Geometry: final body of the model. Coordinates: model frame, mm. Face numbers are marked on the shaded views. A direction names the side the tool comes from. Coordinates: 2 decimals unless noted, no trailing zeros. Order: outer loops, then holes, each group sorted by start corner. A loop starts at its lowest first (then second) coordinate and runs counter-clockwise, first axis right, second up. Notation, with made-up numbers: (2, -32) -> (49, -32) arc R28 cw to (49, -8) -> close; hole circle Ø2 at (-23, 16). An arc over 180 degrees is marked (long way). Answer in a Markdown table with one row per item. Add a question column.
1) Set-up query: the marked faces 1, 2, 3 and 4. Return all of +Z, -Z, +X, -X, +Y, -Y with unobstructed straight access to the full face (end or side cutting, diameter ignored); none if empty.
2) Ray query, line 1 (Y direction, x = -69, z = 3); line 2 (X direction, y = 3.5, z = 5); line 3 (Y direction, x = 51, z = 16.5). Return the intervals inside material, ascending. Write a range as from..to.
3) Pull-direction query (Y, two-part tool) for the marked faces 5, 6 and 7; classes: +Y half, -Y half, draft (parallel to the pull), parting line (faces both ways), or undercut.
4) Section query B-B on y = 44. Return the cut outline in (x, z), then the cut area to 3 significant figures.
5) Contact query for flat-ended pins moving along their axis: P1, Ø1, axis at y = 59.5, z = 9, coming from the +X side; P2, Ø4, axis at y = 3, z = 10.5, coming from the -X side; P3, Ø1.5, axis at x = -21.5, z = 17, coming from the +Y side. Output: stop coordinate, or through.
6) Section query A-A on x = -19. Return the cut outline in (y, z).
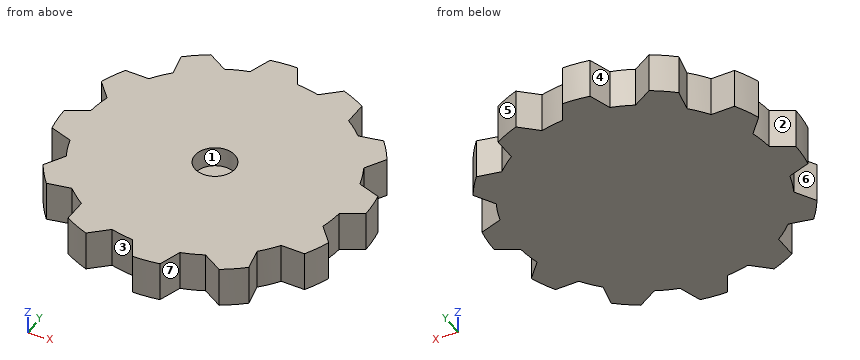
```python
from build123d import *

# Parameters (mm, degrees)
CROQUIS1_R              = 75
SALIENTE_EXTRUIR1_DEPTH = 20
CROQUIS3_R              = 10
CORTAR_EXTRUIR2_DEPTH   = 10
CORTAR_EXTRUIR3_START   = -20
CORTAR_EXTRUIR3_DEPTH   = 20
MATRIZC3_COUNT          = 12


with BuildPart() as part:
    # Croquis1 → Saliente-Extruir1 (new body)
    with BuildSketch(Plane.XY):
        Circle(CROQUIS1_R)
    extrude(amount=SALIENTE_EXTRUIR1_DEPTH)

    # Croquis3 → Cortar-Extruir2 (cut)
    with BuildSketch(Plane.XY.offset(20)):
        Circle(CROQUIS3_R)
    cortar_extruir2 = extrude(amount=-CORTAR_EXTRUIR2_DEPTH, mode=Mode.SUBTRACT)

    # Croquis2 → Cortar-Extruir3 (cut)
    with BuildSketch(Plane.XY.offset(20).offset(CORTAR_EXTRUIR3_START)):
        with BuildLine():
            Line((64.752655376, -5.665123279), (75, 0))
            ThreePointArc((75, 0), (73.860581476, -13.023613325), (70.476946559, -25.651510749))
            Line((70.476946559, -25.651510749), (62.785178709, -16.823237932))
            ThreePointArc((62.785178709, -16.823237932), (64.012503946, -11.287131548), (64.752655376, -5.665123279))
        make_face()
    cortar_extruir3 = extrude(amount=CORTAR_EXTRUIR3_DEPTH, mode=Mode.SUBTRACT)

    # MatrizC3: Cortar-Extruir2, Cortar-Extruir3 ×12 about axis
    matrizc3_axis = Axis((0, 0, 0), (0, 0, 1))
    add([cortar_extruir2.rotate(matrizc3_axis, i * 360 / MATRIZC3_COUNT) for i in range(1, MATRIZC3_COUNT)], mode=Mode.SUBTRACT)
    add([cortar_extruir3.rotate(matrizc3_axis, i * 360 / MATRIZC3_COUNT) for i in range(1, MATRIZC3_COUNT)], mode=Mode.SUBTRACT)


solid = part.part
```
Result:
| question | item | result |
|---|---|---|
| 1 | face 1 | +Z |
| 1 | face 2 | +Z, -Z, -X |
| 1 | face 3 | +Z, -Z, -Y |
| 1 | face 4 | +Z, -Z, +Y |
| 2 | line 1 | -14.69..3.32, 23.96..29.39 |
| 2 | line 2 | -68.67..74.92 |
| 2 | line 3 | -40.3..46.95 |
| 3 | face 5 | +Y half |
| 3 | face 6 | undercut |
| 3 | face 7 | -Y half |
| 4 | outline | (-47.84, 0) -> (60.74, 0) -> (60.74, 20) -> (-47.84, 20) -> close |
| 4 | area | 2,170 mm2 |
| 5 | P1 | x = 37.41 |
| 5 | P2 | x = -73.19 |
| 5 | P3 | y = 61.6 |
| 6 | outline | (-64.68, 0) -> (62.16, 0) -> (62.16, 20) -> (-64.68, 20) -> close |
